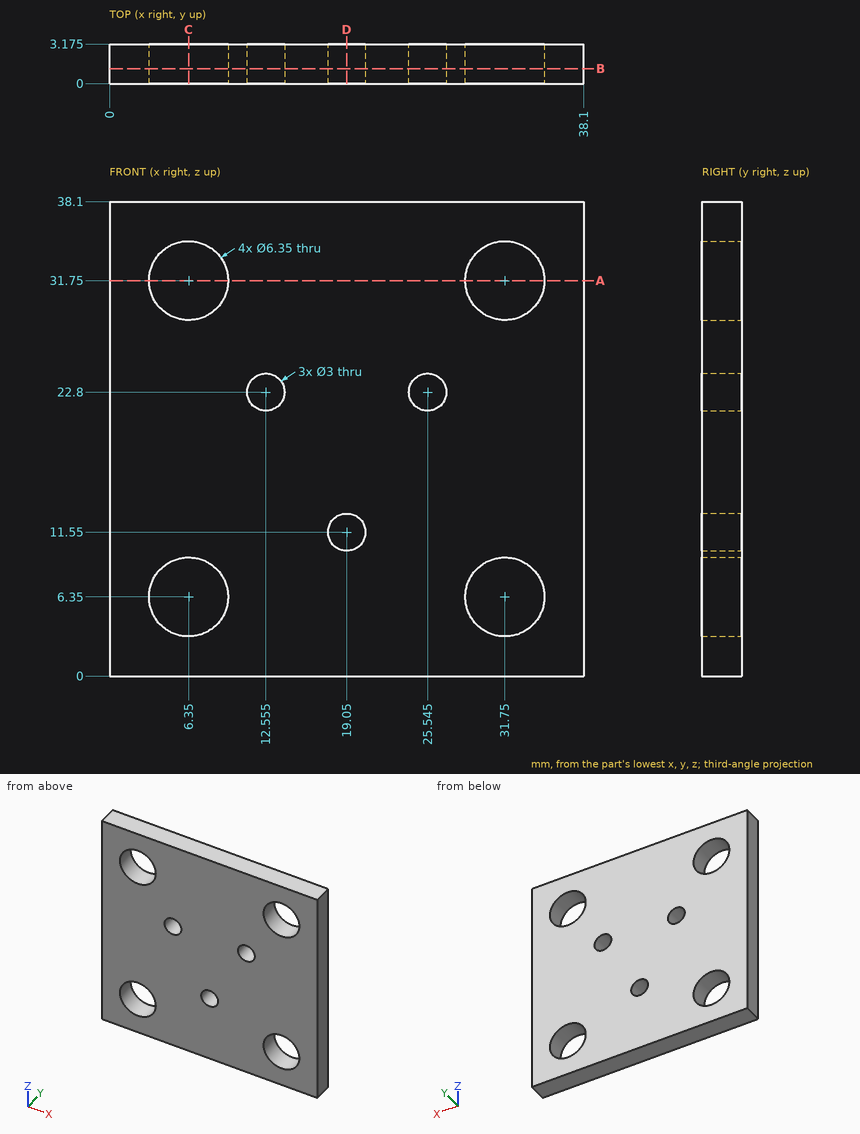
Part print with two shaded views. Sizes in mm from the minimum x, y, z corner. Coordinates: 2 decimals unless noted, no trailing zeros. Write each loop counter-clockwise with the first axis right and the second up, starting at its lowest first coordinate (ties: lowest second). Pieces come first, ordered by that corner, then holes. Notation, with made-up numbers: (-10, 44.25) - (27, 44.25) arc R23 ccw to (27, 60.25) - close; hole circle Ø6 at (25, -26.75). An arc over 180 degrees is marked (long way). Put each result on its own line as item: value.
1. Band-saw the part on D-D (x = 19.05). Write the cut outline in (y, z) (3 decimals).
Final values:
outline: (0, 0) - (3.175, 0) - (3.175, 10.05) - (0, 10.05) - close; (0, 13.05) - (3.175, 13.05) - (3.175, 38.1) - (0, 38.1) - close
2. Band-saw the part on B-B (y = 1.2). Give the number of separate pieces and of enclosed holes in the cut face, then the cut area to 3 significant figures.
Final values:
separate pieces: 1
enclosed holes: 7
area: 1,300 mm²
3. Band-saw the part on A-A (z = 31.75). Write the cut outline in (x, y) (3 decimals).
Final values:
outline: (0, 0) - (3.175, 0) - (3.175, 3.175) - (0, 3.175) - close; (9.525, 0) - (28.575, 0) - (28.575, 3.175) - (9.525, 3.175) - close; (34.925, 0) - (38.1, 0) - (38.1, 3.175) - (34.925, 3.175) - close
4. Band-saw the part on C-C (x = 6.35). Write the cut outline in (y, z) (3 decimals).
Final values:
outline: (0, 0) - (3.175, 0) - (3.175, 3.175) - (0, 3.175) - close; (0, 9.525) - (3.175, 9.525) - (3.175, 28.575) - (0, 28.575) - close; (0, 34.925) - (3.175, 34.925) - (3.175, 38.1) - (0, 38.1) - close
5. Probe line 1 along Z through (x, y) = (31.75, 1.3) (3 decimals); line 2 along X through (y, z) = (1, 22.8) (1 decimal). List the from-to ranges inside material, lowest first. Write a range as [from, to].
Final values:
line 1: z = [0, 3.175], [9.525, 28.575], [34.925, 38.1]
line 2: x = [0, 11.1], [14.1, 24], [27, 38.1]
